Source: CAD feature listing. Evaluate the final solid. Frame: model axes, mm. Round coordinates to 2 decimals unless told otherwise and drop trailing zeros. Order: outer loops, then holes, each group sorted by start corner. A loop starts at its lowest first (then second) coordinate and runs counter-clockwise, first axis right, second up. Notation, with made-up numbers: (-3, 1) - (39, 1) arc R5 ccw to (39, 9) - close; hole circle Ø10 at (-7.5, 4.25). An arc over 180 degrees is marked (long way). Return JSON: item names as keys, results as strings. Group by question number.
1) Section B-B, the plane x = 18. Return loops of the section in (y, z) (3 decimals).
2) Section C-C, the plane y = 5.5. Return loops of the section in (x, z).
3) Section A-A, the plane z = 24. Return loops of the section in (x, y).
4) Contact query for flat-ended pins moving along their axis: P1, Ø1.5, axis at x = 23, z = 20, coming from the -Y side; P2, Ø3, axis at x = 4, z = 8, coming from the -Y side; P3, Ø10, axis at x = 27, z = 9, coming from the +Y side; P4, Ø2.5, axis at y = 19.31, z = 12.06, coming from the +X side. Output: stop coordinate, or through.
5) Section D-D, the plane z = 3. Return loops of the section in (x, y).
6) Ray query, line 1 (Z direction, x = 6.5, y = 19); line 2 (Z direction, x = 17.5, y = 20.5); line 3 (Y direction, x = 7, z = 10). Return the intervals inside material, ascending. Write a range as from..to.
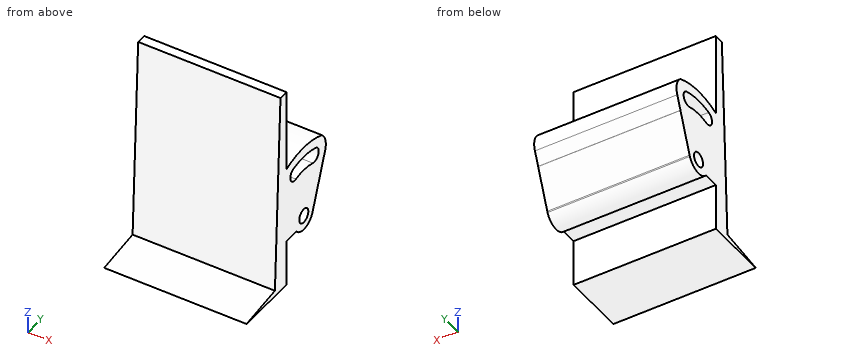
```python
from build123d import *

# Parameters (mm, degrees)
F0_R     = 1.524
F1_DEPTH = 30.48


with BuildPart() as f1:
    # F0 (on Right) → F1 (new body)
    with BuildSketch(Plane.YZ):
        with BuildLine():
            Line((9.577657, 1.260484), (0, 0))
            Line((0, 0), (13.483933, 0))
            Line((13.483933, 0), (13.483933, 10.089966))
            Line((13.483933, 10.089966), (16.819245, 10.089966))
            ThreePointArc((16.819245, 10.089966), (19.740182, 8.919941), (22.233874, 10.83888))
            Line((22.233874, 10.83888), (22.320532, 11.070883))
            Line((22.320532, 11.070883), (25.4, 19.315274))
            Line((25.4, 19.315274), (25.4, 19.366832))
            Line((25.4, 19.366832), (26.482258, 22.212708))
            ThreePointArc((26.482258, 22.212708), (26.623188, 24.560453), (25.4, 26.569328))
            ThreePointArc((25.4, 26.569328), (19.452975, 27.79715), (13.483933, 26.681274))
            Line((13.483933, 26.681274), (13.483933, 44.45))
            Line((13.483933, 44.45), (12.7, 44.45))
            Line((12.7, 44.45), (11.451933, 44.45))
            Line((11.451933, 44.45), (9.577657, 1.260484))
        make_face()
        with Locations((19.305179, 12.065)):
            Circle(F0_R, mode=Mode.SUBTRACT)
        with BuildLine():
            ThreePointArc((15.895544, 25.219289), (19.580856, 25.651203), (23.245615, 25.070149))
            ThreePointArc((23.245615, 25.070149), (24.262218, 23.169709), (22.361779, 22.153106))
            ThreePointArc((22.361779, 22.153106), (19.519022, 22.603831), (16.660322, 22.268794))
            ThreePointArc((16.660322, 22.268794), (14.802685, 23.361652), (15.895544, 25.219289))
        make_face(mode=Mode.SUBTRACT)
    extrude(amount=F1_DEPTH)


solid = f1.part
```
Geometry check:
{
 "1": {"outline": "(0, 0) - (13.484, 0) - (13.484, 10.09) - (16.819, 10.09) arc R3.175 ccw to (22.234, 10.839) - (22.321, 11.071) - (25.4, 19.315) - (25.4, 19.367) - (26.482, 22.213) arc R3.936 ccw to (25.4, 26.569) arc R15.733 ccw to (13.484, 26.681) - (13.484, 44.45) - (11.452, 44.45) - (9.578, 1.26) - close; hole (15.896, 25.219) arc R1.524 ccw to (16.66, 22.269) arc R10.541 cw to (22.362, 22.153) arc R1.524 ccw to (23.246, 25.07) arc R13.589 ccw to start; hole circle Ø3.048 at (19.305, 12.065)"},
 "2": {"outline": "(0, 0) - (30.48, 0) - (30.48, 0.72) - (0, 0.72) - close"},
 "3": {"outline": "(0, 10.56) - (30.48, 10.56) - (30.48, 14.78) - (0, 14.78) - close; (0, 24.28) - (30.48, 24.28) - (30.48, 26.72) - (0, 26.72) - close"},
 "4": {"P1": "y = 10.36", "P2": "y = 9.81", "P3": "y = 23.41", "P4": "through"},
 "5": {"outline": "(0, 9.65) - (30.48, 9.65) - (30.48, 13.48) - (0, 13.48) - close"},
 "6": {"line 1": "8.9..10.57, 13.56..22.6, 25.65..27.79", "line 2": "9.12..11.12, 13.01..22.54, 25.6..27.75", "line 3": "9.96..13.48, 16.89..21.72"}
}
